from build123d import *

# Parameters (mm, degrees)
SKETCH1_W                              = 100
SKETCH1_H                              = 100
SKETCH1_R                              = 25.5
LAMINATION_EXTRUCTION_DEPTH            = 20
SLOT_CUT_DEPTH                         = 74.484692283
SLOT_FILLET_TOP_R                      = 1
SLOT_FILLET_BOTTOM_R                   = 0.5
SLOT_DUPLICATE_COUNT                   = 12
SLOT_FILLET_TOP_OF_SLOT_DUPLICATE_R    = 1
SLOT_FILLET_BOTTOM_OF_SLOT_DUPLICATE_R = 0.5
SKETCH3_R                              = 3.25
BOLT_HOLE_CUT_DEPTH                    = 74.484692283
CORNER_FILLET_R                        = 7
SKETCH4_W                              = 50
SKETCH4_H                              = 100
CUT_EXTRUDE1_DEPTH                     = 74.484692283
SKETCH5_W                              = 50
SKETCH5_H                              = 50
CUT_EXTRUDE2_DEPTH                     = 74.484692283
SKETCH6_R                              = 1.75
CUT_EXTRUDE3_DEPTH                     = 74.484692283
CUT_EXTRUDE4_DEPTH                     = 74.484692283
BOSS_EXTRUDE1_START                    = -20
BOSS_EXTRUDE1_DEPTH                    = 20
FILLET1_R                              = 1


with BuildPart() as part:
    # Sketch1 → Lamination Extruction (new body)
    with BuildSketch(Plane.XY):
        Rectangle(SKETCH1_W, SKETCH1_H)
        Circle(SKETCH1_R, mode=Mode.SUBTRACT)
    extrude(amount=LAMINATION_EXTRUCTION_DEPTH)

    # Sketch2 → Slot Cut (cut, through all)
    with BuildSketch(Plane.XY.offset(20)):
        with BuildLine():
            Line((4.673479277, 28.779136449), (7.75, 40.260868098))
            ThreePointArc((7.75, 40.260868098), (0, 41), (-7.75, 40.260868098))
            Line((-7.75, 40.260868098), (-4.673479277, 28.779136449))
            Line((-4.673479277, 28.779136449), (-1.825, 26.784609787))
            Line((-1.825, 26.784609787), (-1.825, 25.434609787))
            ThreePointArc((-1.825, 25.434609787), (0, 25.5), (1.825, 25.434609787))
            Line((1.825, 25.434609787), (1.825, 26.784609787))
            Line((1.825, 26.784609787), (4.673479277, 28.779136449))
        make_face()
    slot_cut = extrude(amount=-SLOT_CUT_DEPTH, mode=Mode.SUBTRACT)

    # Slot Fillet Top
    slot_fillet_top_edges = [part.edges().sort_by_distance(p)[0] for p in [
        (-7.75, 40.260868098, 10),
        (7.75, 40.260868098, 10),
    ]]
    fillet(slot_fillet_top_edges, radius=SLOT_FILLET_TOP_R)

    # Slot Fillet Bottom
    slot_fillet_bottom_edges = [part.edges().sort_by_distance(p)[0] for p in [
        (4.673479277, 28.779136449, 10),
        (-4.673479277, 28.779136449, 10),
    ]]
    fillet(slot_fillet_bottom_edges, radius=SLOT_FILLET_BOTTOM_R)

    # Slot Duplicate: Slot Cut ×12 about axis
    slot_duplicate_axis = Axis((0, 0, 0), (0, 0, 1))
    for i in range(1, SLOT_DUPLICATE_COUNT):
        add(slot_cut.rotate(slot_duplicate_axis, i * 360 / SLOT_DUPLICATE_COUNT), mode=Mode.SUBTRACT)

    # Slot Fillet Top of Slot Duplicate
    slot_fillet_top_of_slot_duplicate_edges = [part.edges().sort_by_distance(p)[0] for p in [
        (-26.842130928, 30.991934551, 10),
        (-13.41873717, 38.741934551, 10),
        (-38.741934551, 13.41873717, 10),
        (-30.991934551, 26.842130928, 10),
        (-40.260868098, -7.75, 10),
        (-40.260868098, 7.75, 10),
        (-30.991934551, -26.842130928, 10),
        (-38.741934551, -13.41873717, 10),
        (-13.41873717, -38.741934551, 10),
        (-26.842130928, -30.991934551, 10),
        (7.75, -40.260868098, 10),
        (-7.75, -40.260868098, 10),
        (26.842130928, -30.991934551, 10),
        (13.41873717, -38.741934551, 10),
        (38.741934551, -13.41873717, 10),
        (30.991934551, -26.842130928, 10),
        (40.260868098, 7.75, 10),
        (40.260868098, -7.75, 10),
        (30.991934551, 26.842130928, 10),
        (38.741934551, 13.41873717, 10),
        (13.41873717, 38.741934551, 10),
        (26.842130928, 30.991934551, 10),
    ]]
    fillet(slot_fillet_top_of_slot_duplicate_edges, radius=SLOT_FILLET_TOP_OF_SLOT_DUPLICATE_R)

    # Slot Fillet Bottom of Slot Duplicate
    slot_fillet_bottom_of_slot_duplicate_edges = [part.edges().sort_by_distance(p)[0] for p in [
        (-10.342216447, 27.260202902, 10),
        (-18.436920002, 22.586723625, 10),
        (-22.586723625, 18.436920002, 10),
        (-27.260202902, 10.342216447, 10),
        (-28.779136449, 4.673479277, 10),
        (-28.779136449, -4.673479277, 10),
        (-27.260202902, -10.342216447, 10),
        (-22.586723625, -18.436920002, 10),
        (-18.436920002, -22.586723625, 10),
        (-10.342216447, -27.260202902, 10),
        (-4.673479277, -28.779136449, 10),
        (4.673479277, -28.779136449, 10),
        (10.342216447, -27.260202902, 10),
        (18.436920002, -22.586723625, 10),
        (22.586723625, -18.436920002, 10),
        (27.260202902, -10.342216447, 10),
        (28.779136449, -4.673479277, 10),
        (28.779136449, 4.673479277, 10),
        (27.260202902, 10.342216447, 10),
        (22.586723625, 18.436920002, 10),
        (18.436920002, 22.586723625, 10),
        (10.342216447, 27.260202902, 10),
    ]]
    fillet(slot_fillet_bottom_of_slot_duplicate_edges, radius=SLOT_FILLET_BOTTOM_OF_SLOT_DUPLICATE_R)

    # Sketch3 → Bolt Hole Cut (cut, through all)
    with BuildSketch(Plane.XY.offset(20)):
        with Locations((-42.5, 42.5)):
            Circle(SKETCH3_R)
        with Locations((42.5, 42.5)):
            Circle(SKETCH3_R)
        with Locations((42.5, -42.5)):
            Circle(SKETCH3_R)
        with Locations((-42.5, -42.5)):
            Circle(SKETCH3_R)
    extrude(amount=-BOLT_HOLE_CUT_DEPTH, mode=Mode.SUBTRACT)

    # Corner Fillet
    corner_fillet_edges = [part.edges().sort_by_distance(p)[0] for p in [
        (-50, 50, 10),
        (50, 50, 10),
        (50, -50, 10),
        (-50, -50, 10),
    ]]
    fillet(corner_fillet_edges, radius=CORNER_FILLET_R)

    # Sketch4 → Cut-Extrude1 (cut, through all)
    with BuildSketch(Plane.XY.offset(20)):
        with Locations((-25, 0)):
            Rectangle(SKETCH4_W, SKETCH4_H)
    extrude(amount=-CUT_EXTRUDE1_DEPTH, mode=Mode.SUBTRACT)

    # Sketch5 → Cut-Extrude2 (cut, through all)
    with BuildSketch(Plane.XY.offset(20)):
        with Locations((25, 25)):
            Rectangle(SKETCH5_W, SKETCH5_H)
    extrude(amount=-CUT_EXTRUDE2_DEPTH, mode=Mode.SUBTRACT)

    # Sketch6 → Cut-Extrude3 (cut, through all)
    with BuildSketch(Plane.XY.offset(20)):
        with Locations((42.614685392, -14.45643763)):
            Circle(SKETCH6_R)
        with Locations((14.45643763, -42.614685392)):
            Circle(SKETCH6_R)
        with Locations((31.95356776, -31.685477863)):
            Circle(SKETCH6_R)
    extrude(amount=-CUT_EXTRUDE3_DEPTH, mode=Mode.SUBTRACT)

    # Sketch7 → Cut-Extrude4 (cut, through all)
    with BuildSketch(Plane(origin=(0, 0, 0), x_dir=(-1, 0, 0), z_dir=(0, 0, -1))):
        Polygon((-7.468192794, -39.209149287), (-3.721674491, -25.22695263), (0, -25.22695263), (0, -41), align=None)
        Polygon((-39.209149287, -7.468192794), (-25.22695263, -3.721674491), (-25.22695263, 0), (-41, 0), align=None)
    extrude(amount=-CUT_EXTRUDE4_DEPTH, mode=Mode.SUBTRACT)

    # Sketch8 → Boss-Extrude1 (add)
    with BuildSketch(Plane(origin=(0, 0, 0), x_dir=(-1, 0, 0), z_dir=(0, 0, -1)).offset(BOSS_EXTRUDE1_START)):
        with BuildLine():
            Line((-25.22695263, -1.13348404), (-40.660054712, -5.26877128))
            ThreePointArc((-40.660054712, -5.26877128), (-40.914925414, -2.63986333), (-41, 0))
            Line((-41, 0), (-25.22695263, 0))
            Line((-25.22695263, 0), (-25.22695263, -1.13348404))
        make_face()
        with BuildLine():
            Line((0, -41), (0, -25.22695263))
            Line((0, -25.22695263), (-1.13348404, -25.22695263))
            Line((-1.13348404, -25.22695263), (-5.26877128, -40.660054712))
            ThreePointArc((-5.26877128, -40.660054712), (-2.63986333, -40.914925414), (0, -41))
        make_face()
    extrude(amount=BOSS_EXTRUDE1_DEPTH)

    # Fillet1
    fillet1_edges = [part.edges().sort_by_distance(p)[0] for p in [
        (40.660054712, -5.26877128, 10),
        (5.26877128, -40.660054712, 10),
    ]]
    fillet(fillet1_edges, radius=FILLET1_R)


solid = part.part
Here's how the part is built. I have some questions about the finished solid (model axes, mm). A direction names the side the tool comes from. Give positions to 0.01 mm unless a question says otherwise; leave off trailing zeros. Write each loop counter-clockwise with the first axis right and the second up, starting at its lowest first coordinate (ties: lowest second). Pieces come first, ordered by that corner, then holes. Notation, with made-up numbers: (53.5, -10) -> (83.5, -10) arc R26 cw to (83.5, 4) -> close; hole circle Ø10 at (72.25, 37). An arc over 180 degrees is marked (long way). Use one line per item in the form item = value. Start each with the question number.
1. Imagine slicing it at B-B on z = 13.5. State how many separate pieces and enclosed holes the cut face has, plus the area to 3 significant figures.
2. Imagine slicing it at A-A on x = 20. List the corners of the cut face in (y, z) for me.
3. Thinking about a two-plate mould opening in X: for faces 1 (the face through (14.64, -21.71, 10.14)), 2 (the face through (32.41, -3.06, 10.14)), 3 (the face through (38, 0, 10)), which applies, +X half, -X half, draft (parallel to the pull), parting line (faces both ways), or undercut?
4. Will these pins go through, and if not, where does the flat tip stop? pin 1 Ø2 at (y, z) = (-19.5, 5.5) entering from -X; pin 2 Ø1.5 at (y, z) = (-40, 7.5) entering from -X; pin 3 Ø2 at (x, z) = (18.5, 12.5) entering from +Y; pin 4 Ø1.2 at (x, z) = (0.5, 11) entering from +Y.
5. On a 3-axis mill with a long thin cutter (end or side, diameter ignored), from which of +Z, -Z, +X, -X, +Y, -Y can I reach the whole of each face in a straight line? I mean faces 4 (the face through (23.53, -11.48, 10.14)), 5 (the face through (50, -22, 10)), 6 (the face through (40.38, -5.45, 9.86)). Say none if no direction works.
6. If I drill on L1, parallel to Y at x = 42.5, z = 14.5; L2, parallel to Y at x = 39.5, z = 2.75; L3, parallel to X at y = -42, z = 12.25, over which ranges is the centre line in solid material (lowest first)?
Entries:
q1.separate_pieces = 1
q1.enclosed_holes = 4
q1.area = 1,510 mm²
q2.outline = (-50, 0) -> (-35.79, 0) -> (-35.79, 20) -> (-50, 20) -> close; (-24.15, 0) -> (-15.82, 0) -> (-15.82, 20) -> (-24.15, 20) -> close
q3.face_1 = -X half
q3.face_2 = undercut
q3.face_3 = draft
q4.pin_1 = 15.17
q4.pin_2 = 0
q4.pin_3 = -16.43
q4.pin_4 = -25.23
q5.face_4 = +Z, -Z, -X
q5.face_5 = +Z, -Z, +X, +Y, -Y
q5.face_6 = +Z, -Z
q6.L1 = -50 to -45.75, -39.25 to -16.2, -12.71 to 0
q6.L2 = -50 to -43.75, -41.25 to -7.5, -4.96 to 0
q6.L3 = 0 to 12.82, 16.09 to 39.29, 45.71 to 50
